Input: part model. Units: mm. Frame: model coordinates. A direction names the side the tool comes from. Give positions to 0.01 mm unless a question says otherwise; leave off trailing zeros. Write each loop counter-clockwise with the first axis right and the second up, starting at its lowest first coordinate (ties: lowest second). Pieces come first, ordered by that corner, then holes. Notation, with made-up numbers: (83.25, 70) - (93.25, 70) arc R10 cw to (93.25, 75) - close; hole circle Ø8 at (10.25, -27.5). An arc over 180 degrees is marked (long way). Use a Markdown table: item, result. Add a question column.
1. Section query A-A, the plane x = 0. Return loops of the section in (y, z), plus the area to 3 significant figures.
2. Set-up query: faces 1 (the flat face through (0, 200, 0)), 2 (the cylindrical face through (-0.867, 83.81, 3.905)). Return all of +Z, -Z, +X, -X, +Y, -Y with unobstructed straight access to the full face (end or side cutting, diameter ignored); none if empty.
3. Section query B-B, the plane z = 0. Return loops of the section in (x, y), plus the area to 3 significant figures.
4. Pin query (flat end, axial travel): pin 1 (1 mm diameter, centred on x = 19.5, z = 18, fed in from +Y); pin 2 (6 mm diameter, centred on y = 138.5, z = 1.5, fed in from -X); pin 3 (10 mm diameter, centred on x = -20, z = 17.5, fed in from +Y); pin 4 (3 mm diameter, centred on x = 1, z = -15.5, fed in from -Y). Return the tip coordinate at first contact, or that it passes through.
5. Section query C-C, the plane y = 145.5. Return loops of the section in (x, z), plus the area to 3 significant figures.
6. Material intervals for probe 1 along Y at (x, z) = (19, 7.5); probe 2 along Y at (x, z) = (-25.5, -14); probe 3 along X at (y, z) = (157.5, 3), sorted ascending.
```python
from build123d import *

# Parameters (mm, degrees)
SKETCH1_R           = 4
BOSS_EXTRUDE1_DEPTH = 170
SKETCH2_R           = 30
BOSS_EXTRUDE2_DEPTH = 30
FILLET1_R           = 5


with BuildPart() as part:
    # Sketch1 → Boss-Extrude1 (new body)
    with BuildSketch(Plane(origin=(0, 0, 0), x_dir=(1, 0, 0), z_dir=(0, 1, 0))):
        Circle(SKETCH1_R)
    extrude(amount=BOSS_EXTRUDE1_DEPTH)

    # Sketch2 → Boss-Extrude2 (add)
    with BuildSketch(Plane(origin=(0, 170, 0), x_dir=(1, 0, 0), z_dir=(0, 1, 0))):
        Circle(SKETCH2_R)
    extrude(amount=BOSS_EXTRUDE2_DEPTH)

    # Fillet1
    fillet1_edges = [part.edges().sort_by_distance(p)[0] for p in [
        (-30, 170, 0),
        (-30, 200, 0),
    ]]
    fillet(fillet1_edges, radius=FILLET1_R)


solid = part.part
```
Result sheet:
| question | item | result |
|---|---|---|
| 1 | outline | (0, -4) - (170, -4) - (170, -25) arc R5 ccw to (175, -30) - (195, -30) arc R5 ccw to (200, -25) - (200, 25) arc R5 ccw to (195, 30) - (175, 30) arc R5 ccw to (170, 25) - (170, 4) - (0, 4) - close |
| 1 | area | 3,140 mm² |
| 2 | face 1 | +Z, -Z, +X, -X, +Y |
| 2 | face 2 | -Y |
| 3 | outline | (-30, 175) arc R5 ccw to (-25, 170) - (-4, 170) - (-4, 0) - (4, 0) - (4, 170) - (25, 170) arc R5 ccw to (30, 175) - (30, 195) arc R5 ccw to (25, 200) - (-25, 200) arc R5 ccw to (-30, 195) - close |
| 3 | area | 3,140 mm² |
| 4 | pin 1 | stops at y = 199.89 |
| 4 | pin 2 | stops at x = -4 |
| 4 | pin 3 | stops at y = 200 |
| 4 | pin 4 | stops at y = 170 |
| 5 | outline | circle Ø8 at (0, 0) |
| 5 | area | 50.3 mm² |
| 6 | probe 1 | y = 170 to 200 |
| 6 | probe 2 | y = 172.12 to 197.88 |
| 6 | probe 3 | x = -2.65 to 2.65 |
